```python
from build123d import *

# Parameters (mm, degrees)
F2_W     = 5.8
F2_H     = 2
F3_DEPTH = 7
F5_R     = 1.6
F6_REACH = 23.5264833996
F7_SIZE  = 1.5
F8_R     = 1


with BuildPart() as f1:
    # F0 (on Front) → F1 (revolve)
    with BuildSketch(Plane.XZ):
        Polygon((2.55, 10), (2.55, 0), (9, 0), (9, 8), (3.5, 8), (3.5, 10), align=None)
    revolve(axis=Axis((0, 0, 10), (0, 0, 1)))

    # F2 (on face) → F3 (cut)
    with BuildSketch(Plane.XY.offset(8)):
        with Locations((0, 5)):
            Rectangle(F2_W, F2_H)
    extrude(amount=-F3_DEPTH, mode=Mode.SUBTRACT)

    f6_end = f1.faces().sort_by_distance((-2.55, 0, 5))[0]
    # F5 (on offset) → F6 (cut, up to a face of the model that its end follows)
    with BuildSketch(Plane.XZ.offset(-10)):
        with Locations((0, 4)):
            Circle(F5_R)
    f6_long = extrude(amount=F6_REACH, mode=Mode.PRIVATE)
    add(split(f6_long, bisect_by=f6_end, keep=Keep.ALL, mode=Mode.PRIVATE).solids().sort_by_distance((0, 10, 4))[0], mode=Mode.SUBTRACT)

    # F7
    f7_edges = [f1.edges().sort_by_distance(p)[0] for p in [
        (-9, 0, 8),
        (-9, 0, 0),
    ]]
    chamfer(f7_edges, length=F7_SIZE)

    # F8
    f8_edges = [f1.edges().sort_by_distance(p)[0] for p in [
        (-3.5, 0, 8),
    ]]
    fillet(f8_edges, radius=F8_R)


solid = f1.part
```
Check sheet for the modelled part. Datum: model origin and axes. Units: mm. A direction names the side the tool comes from. Coordinates: 2 decimals unless noted, no trailing zeros. Order: outer loops, then holes, each group sorted by start corner. A loop starts at its lowest first (then second) coordinate and runs counter-clockwise, first axis right, second up. Notation, with made-up numbers: (49, 66) -> (105, 66) arc R16 ccw to (105, 97) -> close; hole circle Ø9 at (38.25, 21.25). An arc over 180 degrees is marked (long way). Write each question's results on one line, items separated by ' | '. Start each with the question number.
1) Section check B-B (z = 2). Enter the section's corners in (x, y).
2) Section check C-C (x = 0). Count the separate pieces of the cut face and the enclosed holes in it, and give its area (3 significant figures).
3) Material ranges on line 1 along Y through (x, z) = (0, 6.25); line 2 along Y through (x, z) = (0, 7.75); line 3 along Z through (x, y) = (-1, 4.5), recorded low to high.
4) Depth check by flat-ended pin: pin 1 (1 mm diameter, centred on x = 5.5, z = 4.5, fed in from +Y); pin 2 (0.6 mm diameter, centred on y = 5, z = 3.5, fed in from -X); pin 3 (1.5 mm diameter, centred on y = -5.5, z = 5, fed in from -X). Enter the tip coordinate at first touch or a pass-through.
5) Draft check along X on faces 1 (the face through (-0.46, 3.47, 9.42)), 2 (the face through (0, 5, 1)), 3 (the face through (0, -5, 8)). Enter one of: pulls with the +X half, pulls with the -X half, needs draft (parallel to the pull), parting line crosses it, or undercut.
6) Section check D-D (z = 9.5). Enter the section's corners in (x, y).
7) Section check A-A (y = 0). Enter the section's corners in (x, z).
8) Set-up check for faces 4 (the face through (-1.951, -8.786, 4.035)), 5 (the face through (1.526, 3.231, 4.481)), 6 (the face through (-1.3, 6, 5.3)): record each of +Z, -Z, +X, -X, +Y, -Y from which the full face is reachable in a straight line by a thin tool's end or side.
Checked values:
1) outline: circle Ø18 at (0, 0); hole (-2.9, 4) -> (2.9, 4) -> (2.9, 6) -> (-2.9, 6) -> close; hole circle Ø5.1 at (0, 0)
2) separate pieces: 4 | enclosed holes: 0 | area: 74.6 mm²
3) line 1: -9 to -2.55, 2.55 to 4, 6 to 9 | line 2: -7.75 to -2.55, 2.55 to 4, 6 to 7.75 | line 3: 0 to 1
4) pin 1: y = 7.48 | pin 2: x = -7.68 | pin 3: x = -7.64
5) face 1: parting line crosses it | face 2: undercut | face 3: needs draft
6) outline: circle Ø7 at (0, 0); hole circle Ø5.1 at (0, 0)
7) outline: (-9, 1.5) -> (-7.5, 0) -> (-2.55, 0) -> (-2.55, 10) -> (-3.5, 10) -> (-3.5, 9) arc R1 cw to (-4.5, 8) -> (-7.5, 8) -> (-9, 6.5) -> close; (2.55, 0) -> (7.5, 0) -> (9, 1.5) -> (9, 6.5) -> (7.5, 8) -> (4.5, 8) arc R1 cw to (3.5, 9) -> (3.5, 10) -> (2.55, 10) -> close
8) face 4: +Z, -Z | face 5: +Y | face 6: +Z
